Build history of the part. All positions in model axes, mm. Face numbers are marked on the shaded views. A direction names the side the tool comes from. Give positions to 0.01 mm unless a question says otherwise; leave off trailing zeros. Order: outer loops, then holes, each group sorted by start corner. A loop starts at its lowest first (then second) coordinate and runs counter-clockwise, first axis right, second up. Notation, with made-up numbers: (63, 80.5) -> (82, 80.5) arc R10 ccw to (82, 90.5) -> close; hole circle Ø10 at (37, 60.25). An arc over 180 degrees is marked (long way). One line per question, with ' | ' between items. Start each with the question number.
(1) Drill centre lines: L1, parallel to X at y = 10.5, z = -0.5; L2, parallel to Y at x = 33, z = 20; L3, parallel to X at y = -13, z = -3.5. Where is each one in solid material? Low to high. Write a range as from..to.
(2) Pull direction X, two halves, no side cores. Call the marked faces 6 and 7: +X half, -X half, draft (parallel to the pull), parting line (faces both ways), or undercut.
(3) Cut at C-C (z = -42.5). Give the cut face in (x, y).
(4) Cut at D-D (x = 47.5). Give the cut face in (y, z), then the cut area to 3 significant figures.
(5) Cut at B-B (y = 8). Give the cut face in (x, z), then the cut area to 3 significant figures.
(6) Pin check, flat tips, straight feed: pin 1 Ø5 at (y, z) = (-2.5, 4) entering from -X; pin 2 Ø5 at (x, y) = (139, -22) entering from +Z; pin 3 Ø13 at (x, z) = (15, -43) entering from +Y. Stop position of each tip, or through.
(7) Cut at A-A (x = 250). Give the cut face in (y, z).
(8) Which spindle directions (+Z, -Z, +X, -X, +Y, -Y) get a long thin tool onto all of the face, cutting with end or side? Do the marked faces 1, 2, 3, 4 and 5. Say none if no direction does.
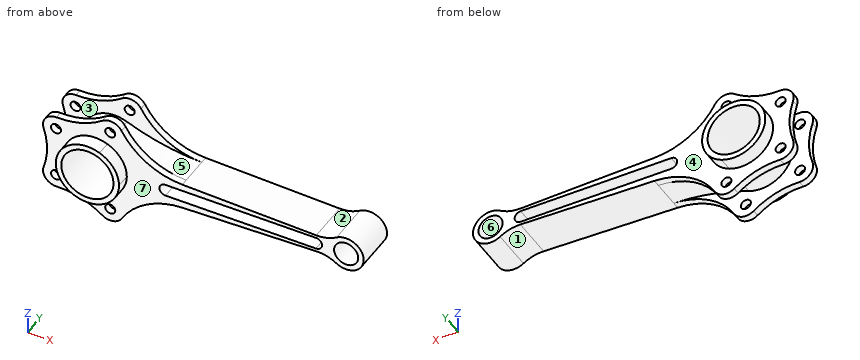
from build123d import *

# Parameters (mm, degrees)
BOSS_EXTRUDE1_DEPTH   = 21
CUT_EXTRUDE1_START    = -14
CUT_EXTRUDE1_DEPTH    = 14
BOSS_EXTRUDE2_START   = -35
BOSS_EXTRUDE2_DEPTH   = 35
SKETCH5_R             = 26
SKETCH5_R_2           = 12
CUT_EXTRUDE2_DEPTH    = 276.530851267
CUT_EXTRUDE3_DEPTH    = 18.5
F_1_0MM_DOWEL_HOLE1_D = 10


# Read off the part's stored shape, not the designer's step: Cut-Extrude1
with BuildPart() as part:
    # Sketch1 → Boss-Extrude1 (new body)
    with BuildSketch(Plane(origin=(0, 0, 0), x_dir=(1, 0, 0), z_dir=(0, 1, 0))):
        with BuildLine():
            Line((86.761016473, 13), (220.287888894, 9))
            ThreePointArc((220.287888894, 9), (230.799852276, 10.288111331), (240.44529895, 14.661435395))
            ThreePointArc((240.44529895, 14.661435395), (267.5, 0), (240.44529895, -14.661435395))
            ThreePointArc((240.44529895, -14.661435395), (230.799852276, -10.288111331), (220.287888894, -9))
            Line((220.287888894, -9), (86.761016473, -13))
            ThreePointArc((86.761016473, -13), (51.764556155, -23.293555937), (26.304940485, -49.418591795))
            ThreePointArc((26.304940485, -49.418591795), (17.645869205, -55.727897554), (7.189691393, -53.392260556))
            ThreePointArc((7.189691393, -53.392260556), (-14.44681941, -42.272249892), (-38.551485077, -38.992260556))
            ThreePointArc((-38.551485077, -38.992260556), (-49.370923708, -33.838618593), (-51.376901133, -22.023529412))
            ThreePointArc((-51.376901133, -22.023529412), (-47.925892025, 0), (-51.376901133, 22.023529412))
            ThreePointArc((-51.376901133, 22.023529412), (-49.370923708, 33.838618593), (-38.551485077, 38.992260556))
            ThreePointArc((-38.551485077, 38.992260556), (-14.44681941, 42.272249892), (7.189691393, 53.392260556))
            ThreePointArc((7.189691393, 53.392260556), (17.645869205, 55.727897554), (26.304940485, 49.418591795))
            ThreePointArc((26.304940485, 49.418591795), (51.764556155, 23.293555937), (86.761016473, 13))
        make_face()
    extrude(amount=BOSS_EXTRUDE1_DEPTH)

    # Cut-Extrude1 outline → Cut-Extrude1 (cut)
    with BuildSketch(Plane.XZ.offset(CUT_EXTRUDE1_START)):
        with BuildLine():
            ThreePointArc((86.761016473, -13), (48.697663607, -17.630477543), (12.103585769, -29.081836454))
            ThreePointArc((12.103585769, -29.081836454), (-31.5, 0), (12.103585769, 29.081836454))
            ThreePointArc((12.103585769, 29.081836454), (48.697663607, 17.630477543), (86.761016473, 13))
            ThreePointArc((86.761016473, 13), (51.764556155, 23.293555937), (26.304940485, 49.418591795))
            ThreePointArc((26.304940485, 49.418591795), (17.645869204, 55.727897554), (7.189691393, 53.392260556))
            ThreePointArc((7.189691393, 53.392260556), (-14.446819411, 42.272249892), (-38.551485077, 38.992260556))
            ThreePointArc((-38.551485077, 38.992260556), (-49.370923708, 33.838618593), (-51.376901133, 22.023529412))
            ThreePointArc((-51.376901133, 22.023529412), (-47.925892025, 0), (-51.376901133, -22.023529412))
            ThreePointArc((-51.376901133, -22.023529412), (-49.370923708, -33.838618593), (-38.551485077, -38.992260556))
            ThreePointArc((-38.551485077, -38.992260556), (-14.446819411, -42.272249892), (7.189691393, -53.392260556))
            ThreePointArc((7.189691393, -53.392260556), (17.645869204, -55.727897554), (26.304940485, -49.418591795))
            ThreePointArc((26.304940485, -49.418591795), (51.764556155, -23.293555937), (86.761016473, -13))
        make_face()
    extrude(amount=CUT_EXTRUDE1_DEPTH, mode=Mode.SUBTRACT)

    # Sketch3 → Boss-Extrude2 (add)
    with BuildSketch(Plane.XZ.offset(BOSS_EXTRUDE2_START)):
        with BuildLine():
            ThreePointArc((12.103585769, -29.081836454), (26.20603892, -17.47837304), (31.5, 0))
            ThreePointArc((31.5, 0), (26.20603892, 17.47837304), (12.103585769, 29.081836454))
            ThreePointArc((12.103585769, 29.081836454), (-31.5, 0), (12.103585769, -29.081836454))
        make_face()
    extrude(amount=BOSS_EXTRUDE2_DEPTH)

    # Sketch5 → Cut-Extrude2 (cut, through all)
    with BuildSketch(Plane(origin=(0, 35, 0), x_dir=(1, 0, 0), z_dir=(0, 1, 0))):
        with Locations(Location((0, 0, 0), (0, 0, 270))):
            Circle(SKETCH5_R)
        with Locations(Location((250, 0, 0), (0, 0, 270))):
            Circle(SKETCH5_R_2)
    extrude(amount=-CUT_EXTRUDE2_DEPTH, mode=Mode.SUBTRACT)

    # Sketch6 → Cut-Extrude3 (cut)
    with BuildSketch(Plane(origin=(0, 21, 0), x_dir=(1, 0, 0), z_dir=(0, 1, 0))):
        with BuildLine():
            Line((70, 6), (220, 6))
            ThreePointArc((220, 6), (226, 0), (220, -6))
            Line((220, -6), (70, -6))
            ThreePointArc((70, -6), (64, 0), (70, 6))
        make_face()
    extrude(amount=-CUT_EXTRUDE3_DEPTH, mode=Mode.SUBTRACT)

    # Ø1.0mm Dowel Hole1 (through all)
    with Locations(Plane(origin=(15, 21, 43), x_dir=(0, 0, 1), z_dir=(0, 1, 0))):
        with Locations((0, 0)):
            f_1_0mm_dowel_hole1 = Hole(F_1_0MM_DOWEL_HOLE1_D / 2)

    # Sketch-Pattern1: Ø1.0mm Dowel Hole1 at 3 more places
    with Locations((-54, 0, -69), (-54, 0, -17), (0, 0, -86)):
        add(f_1_0mm_dowel_hole1, mode=Mode.SUBTRACT)

    # Mirror1: part across plane


with BuildPart() as part_1:
    add(part.part)
    add(part.part.mirror(Plane(origin=(-39, 0, -26), x_dir=(0, 0, 1), z_dir=(0, -1, 0))))


solid = part_1.part
Result set:
1) L1: x = -31.5..-26, 26..64.02, 225.98..238.01, 261.99..267.49 | L2: y = -21..21 | L3: x = -31.3..-25.76, 25.76..65.13, 224.87..238.52, 261.48..267.15
2) face 6: undercut | face 7: draft
3) outline: (-13.74, -21) -> (10.03, -21) -> (10.03, -14) -> (-13.74, -14) -> close; (-13.74, 14) -> (10.03, 14) -> (10.03, 21) -> (-13.74, 21) -> close; (19.97, -21) -> (30.77, -21) -> (30.77, -14) -> (19.97, -14) -> close; (19.97, 14) -> (30.77, 14) -> (30.77, 21) -> (19.97, 21) -> close
4) outline: (-21, -26.07) -> (-14, -26.07) -> (-14, -17.89) -> (14, -17.89) -> (14, -26.07) -> (21, -26.07) -> (21, 26.07) -> (14, 26.07) -> (14, 17.89) -> (-14, 17.89) -> (-14, 26.07) -> (-21, 26.07) -> close | area: 1,730 mm2
5) outline: (12.1, -29.08) arc R210.72 cw to (86.76, -13) -> (220.29, -9) arc R35 cw to (240.45, -14.66) arc R17.5 ccw (long way) to (240.45, 14.66) arc R35 cw to (220.29, 9) -> (86.76, 13) arc R210.72 cw to (12.1, 29.08) arc R31.5 ccw (long way) to start; hole circle Ø52 at (0, 0); hole (70, -6) -> (220, -6) arc R6 ccw to (220, 6) -> (70, 6) arc R6 ccw to start; hole circle Ø24 at (250, 0) | area: 4,770 mm2
6) pin 1: stops at x = -31.46 | pin 2: stops at z = 11.5 | pin 3: stops at y = 21
7) outline: (-21, -17.5) -> (21, -17.5) -> (21, -12) -> (-21, -12) -> close; (-21, 12) -> (21, 12) -> (21, 17.5) -> (-21, 17.5) -> close
8) face 1: -Z, +Y, -Y | face 2: +Z, +Y, -Y | face 3: none | face 4: +Y | face 5: +Z
